```python
from build123d import *

# Parameters (mm, degrees)
IZIM1_R                     = 55
Y_KSEKLIK_EKSTR_ZYON1_DEPTH = 11
IZIM2_OUTSIDE_W             = 143.422
IZIM2_OUTSIDE_H             = 143.422
IZIM2_OUTSIDE_R             = 47.5
KES_EKSTR_ZYON1_DEPTH       = 14.5
IZIM3_R                     = 1.55
KES_EKSTR_ZYON2_DEPTH       = 80.121741639
DAIRESEL_KAPLAMA1_COUNT     = 8
IZIM4_R                     = 39.875
KES_EKSTR_ZYON3_DEPTH       = 81.833161512
IZIM5_R                     = 47.5
IZIM5_R_2                   = 39.875
Y_KSEKLIK_EKSTR_ZYON2_DEPTH = 95.5


with BuildPart() as part:
    # Çizim1 → Yükseklik-Ekstrüzyon1 (new, symmetric)
    with BuildSketch(Plane.XY):
        Circle(IZIM1_R)
    extrude(amount=Y_KSEKLIK_EKSTR_ZYON1_DEPTH, both=True)

    # Çizim2 outside → Kes-Ekstrüzyon1 (cut)
    with BuildSketch(Plane(origin=(0, 0, -11), x_dir=(-1, 0, 0), z_dir=(0, 0, -1))):
        Rectangle(IZIM2_OUTSIDE_W, IZIM2_OUTSIDE_H)
        Circle(IZIM2_OUTSIDE_R, mode=Mode.SUBTRACT)
    extrude(amount=-KES_EKSTR_ZYON1_DEPTH, mode=Mode.SUBTRACT)

    # Çizim3 → Kes-Ekstrüzyon2 (cut, through all)
    with BuildSketch(Plane(origin=(0, 0, 3.5), x_dir=(-1, 0, 0), z_dir=(0, 0, -1))):
        with Locations((0, 51.25)):
            Circle(IZIM3_R)
    kes_ekstr_zyon2 = extrude(amount=-KES_EKSTR_ZYON2_DEPTH, mode=Mode.SUBTRACT)

    # Dairesel Kaplama1: Kes-Ekstrüzyon2 ×8 about axis
    dairesel_kaplama1_axis = Axis((0, 0, 0), (0, 0, 1))
    for i in range(1, DAIRESEL_KAPLAMA1_COUNT):
        add(kes_ekstr_zyon2.rotate(dairesel_kaplama1_axis, i * 360 / DAIRESEL_KAPLAMA1_COUNT), mode=Mode.SUBTRACT)

    # Çizim4 → Kes-Ekstrüzyon3 (cut, through all)
    with BuildSketch(Plane.XY.offset(11)):
        Circle(IZIM4_R)
    extrude(amount=-KES_EKSTR_ZYON3_DEPTH, mode=Mode.SUBTRACT)

    # Çizim5 → Yükseklik-Ekstrüzyon2 (add)
    with BuildSketch(Plane(origin=(0, 0, -11), x_dir=(-1, 0, 0), z_dir=(0, 0, -1))):
        Circle(IZIM5_R)
        with Locations(Location((0, 0, 0), (0, 0, 180))):
            Circle(IZIM5_R_2, mode=Mode.SUBTRACT)
    extrude(amount=Y_KSEKLIK_EKSTR_ZYON2_DEPTH)


solid = part.part
```
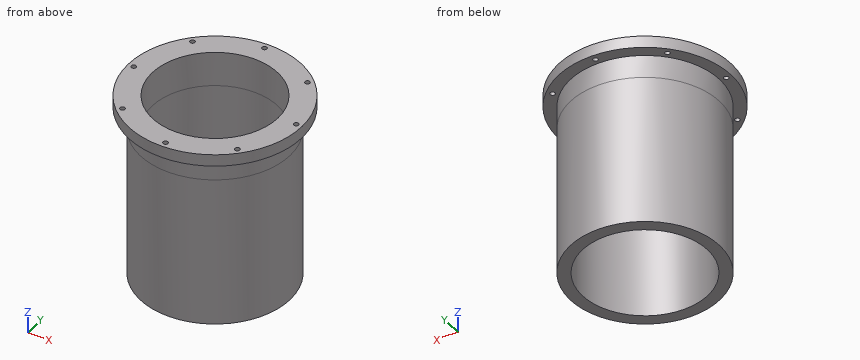
Build history of the part. All positions in model axes, mm. Give positions to 0.01 mm unless a question says otherwise; leave off trailing zeros. Loops run counter-clockwise (first coordinate to the right, second up) from the corner with the lowest first, then second, coordinate; pieces in that order, holes last.
1) Probe line 1 along Y through (x, z) = (0, 6) (3 decimals); line 2 along Y through (x, z) = (29, -44); line 3 along X through (y, z) = (-21.5, -65). List the from-to ranges inside material, lowest first.
Values follow:
line 1: y = -55 to -52.8, -49.7 to -39.875, 39.875 to 49.7, 52.8 to 55
line 2: y = -37.62 to -27.37, 27.37 to 37.62
line 3: x = -42.36 to -33.58, 33.58 to 42.36
2) Band-saw the part on C-C on z = -64. List the corners of the cut face in (x, y) (3 decimals), then the cut area to 3 significant figures.
Values follow:
outline: circle Ø95 at (0, 0); hole circle Ø79.75 at (0, 0)
area: 2,090 mm2
3) Drop flat-ended pins along their axis: P1, Ø2, axis at x = -21, z = -48, coming from the -Y side; P2, Ø3.5, axis at x = -36.24, y = 36.24, coming from the -Z side; P3, Ø1.9, axis at x = 0, y = 51.25, coming from the +Z side; P4, Ø4, axis at x = 35.5, z = -44.5, coming from the +Y side. Give the stop position or say it passes through.
Values follow:
P1: stops at y = -43.08
P2: stops at z = 3.5
P3: passes through
P4: stops at y = 33.67
4) Band-saw the part on A-A on y = -11. List the corners of the cut face in (x, z), then the cut area to 3 significant figures.
Values follow:
outline: (-53.89, 3.5) - (-46.21, 3.5) - (-46.21, -106.5) - (-38.33, -106.5) - (-38.33, 11) - (-53.89, 11) - close; (38.33, -106.5) - (46.21, -106.5) - (46.21, 3.5) - (53.89, 3.5) - (53.89, 11) - (38.33, 11) - close
area: 1,970 mm2
5) Band-saw the part on B-B on x = 29. List the corners of the cut face in (y, z).
Values follow:
outline: (-46.73, 3.5) - (-37.62, 3.5) - (-37.62, -106.5) - (-27.37, -106.5) - (-27.37, 11) - (-46.73, 11) - close; (27.37, -106.5) - (37.62, -106.5) - (37.62, 3.5) - (46.73, 3.5) - (46.73, 11) - (27.37, 11) - close
